from build123d import *

# Parameters (mm, degrees)
SKETCH014_W     = 9
SKETCH014_H     = 15
PAD004_DEPTH    = 2
SKETCH015_R     = 1.65
POCKET009_DEPTH = 1
SKETCH016_R     = 0.95
POCKET010_DEPTH = 5
SKETCH017_W     = 1
SKETCH017_H     = 8.8
PAD005_DEPTH    = 3.9
SKETCH018_R     = 0.6
POCKET011_DEPTH = 5
CHAMFER_SIZE    = 1


with BuildPart() as part:
    # Sketch014 → Pad004 (new body)
    with BuildSketch(Plane.XY):
        with Locations((0, -5.5)):
            Rectangle(SKETCH014_W, SKETCH014_H)
    extrude(amount=PAD004_DEPTH)

    # Sketch015 (on Face18 of Pad003) → Pocket009 (cut)
    with BuildSketch(Plane(origin=(0, 0, 0), x_dir=(1, 0, 0), z_dir=(0, 0, -1))):
        Circle(SKETCH015_R)
    extrude(amount=-POCKET009_DEPTH, mode=Mode.SUBTRACT)

    # Sketch016 (on Face18 of Pad003) → Pocket010 (cut)
    with BuildSketch(Plane(origin=(0, 0, 0.5), x_dir=(1, 0, 0), z_dir=(0, 0, -1))):
        Circle(SKETCH016_R)
    extrude(amount=-POCKET010_DEPTH, mode=Mode.SUBTRACT)

    # Sketch017 → Pad005 (join)
    with BuildSketch(Plane.XY.offset(2)):
        with Locations((-4, -6.5)):
            Rectangle(SKETCH017_W, SKETCH017_H)
        with Locations((4, -6.5)):
            Rectangle(SKETCH017_W, SKETCH017_H)
    extrude(amount=PAD005_DEPTH)

    # Sketch018 → Pocket011 (cut)
    with BuildSketch(Plane(origin=(0, -7.58, 0), x_dir=(1, 0, 0), z_dir=(0, 0, 1))):
        with Locations((-1.28, 1.28)):
            Circle(SKETCH018_R)
        with Locations((1.291315, 1.272746)):
            Circle(SKETCH018_R)
        with Locations((-1.28, -1.28)):
            Circle(SKETCH018_R)
        with Locations((1.28, -1.28)):
            Circle(SKETCH018_R)
    extrude(amount=POCKET011_DEPTH, mode=Mode.SUBTRACT)

    # Chamfer
    chamfer_edges = [part.edges().sort_by_distance(p)[0] for p in [
        (0, -13, 0),
    ]]
    chamfer(chamfer_edges, length=CHAMFER_SIZE)


with BuildPart() as part_1:
    # Body002 placement: moved
    add(part.part.moved(Location((0, 0, -9.5))))


solid = part_1.part
Can you work these out from the model? Positions are in its coordinate system, mm. A direction names the side the tool comes from. Round coordinates to 2 decimals unless told otherwise and drop trailing zeros. Loops run counter-clockwise (first coordinate to the right, second up) from the corner with the lowest first, then second, coordinate; pieces in that order, holes last. Notation, with made-up numbers: (-24.5, 69.5) - (17.5, 69.5) arc R16 cw to (17.5, 92.5) - close; hole circle Ø6 at (34.5, -11). An arc over 180 degrees is marked (long way). Answer in a Markdown table with one row per item. Add a question column.
Q1. I want a section at A-A on z = -5. List the corners of the cut face in (x, y) for me, and give its area (3 significant figures).
Q2. For pin 1 Ø1.1 at (x, z) = (4, -5) entering from -Y; pin 2 Ø1.5 at (x, y) = (-2, -4.5) entering from +Z; pin 3 Ø0.8 at (x, z) = (-4, -6) entering from +Y, each with a flat end and sliding along its axis, tell me the tip position at first contact or that it passes through.
Q3. I want a section at C-C on x = 1.28. List the corners of the cut face in (y, z) for me, and give its area (3 significant figures).
Q4. Which directions (+Z, -Z, +X, -X, +Y, -Y) give clear straight access to the entire face, cutting with the end or side of a thin tool? Please do faces 4 (the flat face through (0, -13, -8)), 5 (the cylindrical face through (-1.216, -1.115, -9.007)), 6 (the flat face through (-0.1, -12.5, -9)), 7 (the flat face through (-3.5, -7, -6)), 8 (the flat face through (4, -10.9, -6)).
Q5. I need wall thicknesses on L1, parallel to Y at x = -1.28, z = -8.45; L2, parallel to X at y = -9, z = -6.85; L3, parallel to X at y = 0, z = -9.1. Which ranges of each line are inside material? Lowest first, please.
Q6. I want a section at B-B on y = 0. List the corners of the cut face in (x, z) for me.
Q7. We'd pull the mould along X, two halves only. Please class faces 1 (the flat face through (1, 1, -8.5)), 2 (the flat face through (0, 2, -9)), 3 (the flat face through (4.5, -6, -7)): pulls with the +X half, pulls with the -X half, needs draft (parallel to the pull), parting line crosses it, or undercut.
Q8. I want a section at D-D on y = -8.86. List the corners of the cut face in (x, z) for me, and give its area (3 significant figures).
A:
| question | item | result |
|---|---|---|
| 1 | outline | (-4.5, -10.9) - (-3.5, -10.9) - (-3.5, -2.1) - (-4.5, -2.1) - close; (3.5, -10.9) - (4.5, -10.9) - (4.5, -2.1) - (3.5, -2.1) - close |
| 1 | area | 17.6 mm^2 |
| 2 | pin 1 | y = -10.9 |
| 2 | pin 2 | z = -7.5 |
| 2 | pin 3 | y = -2.1 |
| 3 | outline | (-13, -8.5) - (-12, -9.5) - (-9.46, -9.5) - (-9.46, -7.5) - (-13, -7.5) - close; (-8.26, -9.5) - (-6.91, -9.5) - (-6.91, -7.5) - (-8.26, -7.5) - close; (-5.71, -9.5) - (-1.04, -9.5) - (-1.04, -8.5) - (1.04, -8.5) - (1.04, -9.5) - (2, -9.5) - (2, -7.5) - (-5.71, -7.5) - close |
| 3 | area | 22.6 mm^2 |
| 4 | face 4 | +Z, -Z, +X, -X, -Y |
| 4 | face 5 | -Z |
| 4 | face 6 | -Z, +X, -X, -Y |
| 4 | face 7 | +Z, +Y, -Y |
| 4 | face 8 | +Z, +X, -X, -Y |
| 5 | L1 | -13 to -9.46, -8.26 to -6.9, -5.7 to 2 |
| 5 | L2 | -4.5 to -3.5, 3.5 to 4.5 |
| 5 | L3 | -4.5 to -1.65, 1.65 to 4.5 |
| 6 | outline | (-4.5, -9.5) - (-1.65, -9.5) - (-1.65, -8.5) - (-0.95, -8.5) - (-0.95, -7.5) - (-4.5, -7.5) - close; (0.95, -8.5) - (1.65, -8.5) - (1.65, -9.5) - (4.5, -9.5) - (4.5, -7.5) - (0.95, -7.5) - close |
| 7 | face 1 | undercut |
| 7 | face 2 | needs draft |
| 7 | face 3 | pulls with the +X half |
| 8 | outline | (-4.5, -9.5) - (-1.88, -9.5) - (-1.88, -7.5) - (-3.5, -7.5) - (-3.5, -3.6) - (-4.5, -3.6) - close; (-0.68, -9.5) - (0.68, -9.5) - (0.68, -7.5) - (-0.68, -7.5) - close; (1.88, -9.5) - (4.5, -9.5) - (4.5, -3.6) - (3.5, -3.6) - (3.5, -7.5) - (1.88, -7.5) - close |
| 8 | area | 21.0 mm^2 |
